Input: part model. Units: mm. Frame: model coordinates. Face numbers are marked on the shaded views. A direction names the side the tool comes from. Give positions to 0.01 mm unless a question says otherwise; leave off trailing zeros. Loops run counter-clockwise (first coordinate to the right, second up) from the corner with the lowest first, then second, coordinate; pieces in that order, holes last. Notation, with made-up numbers: (38.25, 3.25) - (43.25, 3.25) arc R16 ccw to (43.25, 14.25) - close; hole circle Ø5 at (39.25, 7). An arc over 180 degrees is marked (long way). One line per item, written item: value.
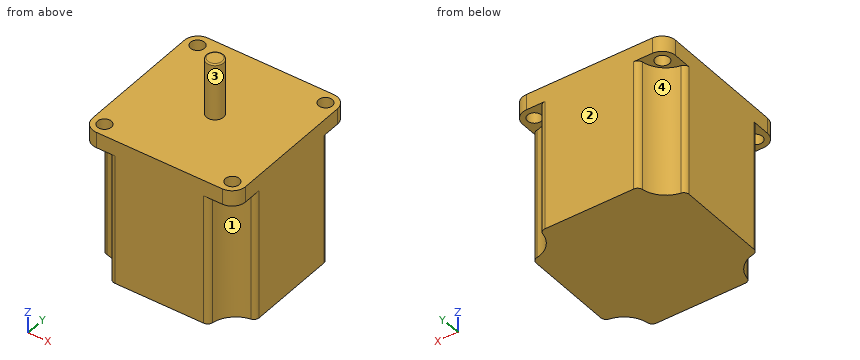
from build123d import *

# Parameters (mm, degrees)
ESQUISSE2_W             = 56.4
ESQUISSE2_H             = 56.4
BOSS_EXTRU_2_DEPTH      = 54
ESQUISSE3_R             = 2.55
ENL_V_MAT_EXTRU_1_DEPTH = 54
CONG_2_R                = 5
CONG_3_R                = 5
CONG_4_R                = 5
CONG_6_R                = 5
ESQUISSE4_R             = 2.55
ENL_V_MAT_EXTRU_2_DEPTH = 48.2
CONG_7_R                = 2
CONG_8_R                = 2
CONG_9_R                = 2
CONG_10_R               = 2
CONG_11_R               = 2
CONG_12_R               = 2
CONG_13_R               = 2
CONG_14_R               = 2
ESQUISSE5_R             = 3.175
BOSS_EXTRU_3_DEPTH      = 21
CONG_15_R               = 0.5


with BuildPart() as part:
    # Esquisse2 → Boss.-Extru.2 (new body)
    with BuildSketch(Plane.XY):
        Rectangle(ESQUISSE2_W, ESQUISSE2_H)
    extrude(amount=BOSS_EXTRU_2_DEPTH)

    # Esquisse3 → Enlèv. mat.-Extru.1 (cut)
    with BuildSketch(Plane.XY.offset(54)):
        with Locations((-23.57, 23.57)):
            Circle(ESQUISSE3_R)
        with Locations((23.57, 23.57)):
            Circle(ESQUISSE3_R)
        with Locations((23.57, -23.57)):
            Circle(ESQUISSE3_R)
        with Locations((-23.57, -23.57)):
            Circle(ESQUISSE3_R)
    extrude(amount=-ENL_V_MAT_EXTRU_1_DEPTH, mode=Mode.SUBTRACT)

    # Congé2
    cong_2_edges = [part.edges().sort_by_distance(p)[0] for p in [
        (28.2, 28.2, 27),
    ]]
    fillet(cong_2_edges, radius=CONG_2_R)

    # Congé3
    cong_3_edges = [part.edges().sort_by_distance(p)[0] for p in [
        (28.2, -28.2, 27),
    ]]
    fillet(cong_3_edges, radius=CONG_3_R)

    # Congé4
    cong_4_edges = [part.edges().sort_by_distance(p)[0] for p in [
        (-28.2, 28.2, 27),
    ]]
    fillet(cong_4_edges, radius=CONG_4_R)

    # Congé6
    cong_6_edges = [part.edges().sort_by_distance(p)[0] for p in [
        (-28.2, -28.2, 27),
    ]]
    fillet(cong_6_edges, radius=CONG_6_R)

    # Esquisse4 → Enlèv. mat.-Extru.2 (cut)
    with BuildSketch(Plane(origin=(0, 0, 0), x_dir=(-1, 0, 0), z_dir=(0, 0, -1))):
        with BuildLine():
            ThreePointArc((-18.2, -28.2), (-21.128932188, -21.128932188), (-28.2, -18.2))
            Line((-28.2, -18.2), (-28.2, -23.2))
            ThreePointArc((-28.2, -23.2), (-26.735533906, -26.735533906), (-23.2, -28.2))
            Line((-23.2, -28.2), (-18.2, -28.2))
        make_face()
        with Locations((-23.57, -23.57)):
            Circle(ESQUISSE4_R, mode=Mode.SUBTRACT)
        with BuildLine():
            Line((-28.2, 28.2), (-18.2, 28.2))
            ThreePointArc((-18.2, 28.2), (-21.128932188, 21.128932188), (-28.2, 18.2))
            Line((-28.2, 18.2), (-28.2, 28.2))
        make_face()
        with BuildLine():
            ThreePointArc((28.2, -18.2), (21.128932188, -21.128932188), (18.2, -28.2))
            Line((18.2, -28.2), (28.2, -28.2))
            Line((28.2, -28.2), (28.2, -18.2))
        make_face()
        with BuildLine():
            ThreePointArc((18.2, 28.2), (21.128932188, 21.128932188), (28.2, 18.2))
            Line((28.2, 18.2), (28.2, 28.2))
            Line((28.2, 28.2), (18.2, 28.2))
        make_face()
    extrude(amount=-ENL_V_MAT_EXTRU_2_DEPTH, mode=Mode.SUBTRACT)

    # Congé7
    cong_7_edges = [part.edges().sort_by_distance(p)[0] for p in [
        (18.2, 28.2, 24.1),
    ]]
    fillet(cong_7_edges, radius=CONG_7_R)

    # Congé8
    cong_8_edges = [part.edges().sort_by_distance(p)[0] for p in [
        (28.2, 18.2, 24.1),
    ]]
    fillet(cong_8_edges, radius=CONG_8_R)

    # Congé9
    cong_9_edges = [part.edges().sort_by_distance(p)[0] for p in [
        (-18.2, 28.2, 24.1),
    ]]
    fillet(cong_9_edges, radius=CONG_9_R)

    # Congé10
    cong_10_edges = [part.edges().sort_by_distance(p)[0] for p in [
        (-28.2, 18.2, 24.1),
    ]]
    fillet(cong_10_edges, radius=CONG_10_R)

    # Congé11
    cong_11_edges = [part.edges().sort_by_distance(p)[0] for p in [
        (-28.2, -18.2, 24.1),
    ]]
    fillet(cong_11_edges, radius=CONG_11_R)

    # Congé12
    cong_12_edges = [part.edges().sort_by_distance(p)[0] for p in [
        (-18.2, -28.2, 24.1),
    ]]
    fillet(cong_12_edges, radius=CONG_12_R)

    # Congé13
    cong_13_edges = [part.edges().sort_by_distance(p)[0] for p in [
        (18.2, -28.2, 24.1),
    ]]
    fillet(cong_13_edges, radius=CONG_13_R)

    # Congé14
    cong_14_edges = [part.edges().sort_by_distance(p)[0] for p in [
        (28.2, -18.2, 24.1),
    ]]
    fillet(cong_14_edges, radius=CONG_14_R)

    # Esquisse5 → Boss.-Extru.3 (add)
    with BuildSketch(Plane.XY.offset(54)):
        Circle(ESQUISSE5_R)
    extrude(amount=BOSS_EXTRU_3_DEPTH)

    # Congé15
    cong_15_edges = [part.edges().sort_by_distance(p)[0] for p in [
        (-3.175, 0, 75),
    ]]
    fillet(cong_15_edges, radius=CONG_15_R)


solid = part.part
Item 1: Access query for the marked faces 1, 2, 3 and 4. Directions: +Z, -Z, +X, -X, +Y, -Y. A direction counts if a zero-diameter tool reaches every point of the face in a straight line with its end or side. Return the directions, or none.
Verdict:
face 1: -Z, +X, -Y
face 2: +Z, -Z, +X, -X, +Y
face 3: +Z
face 4: -Z, -X, +Y
Item 2: Pin query (flat end, axial travel): P1, Ø3.5, axis at x = 23, y = 24.5, coming from the -Z side; P2, Ø5, axis at x = -17, y = -19, coming from the +Z side; P3, Ø3, axis at x = -23.57, y = 23.57, coming from the -Z side; P4, Ø5, axis at x = -4, z = 66, coming from the +Y side. Return the tip coordinate at first contact, or that it passes through.
Verdict:
P1: stops at z = 48.2
P2: stops at z = 54
P3: passes through
P4: stops at y = 2.8
Item 3: Section D-D, the plane x = 5.5. Output: boundary loops of the cut face in (y, z).
Verdict:
outline: (-28.2, 0) - (28.2, 0) - (28.2, 54) - (-28.2, 54) - close
Item 4: Section A-A, the plane z = 53. Output: boundary loops of the cut face in (x, y).
Verdict:
outline: (-28.2, -23.2) arc R5 ccw to (-23.2, -28.2) - (23.2, -28.2) arc R5 ccw to (28.2, -23.2) - (28.2, 23.2) arc R5 ccw to (23.2, 28.2) - (-23.2, 28.2) arc R5 ccw to (-28.2, 23.2) - close; hole circle Ø5.1 at (-23.57, -23.57); hole circle Ø5.1 at (-23.57, 23.57); hole circle Ø5.1 at (23.57, -23.57); hole circle Ø5.1 at (23.57, 23.57)
Item 5: Section B-B, the plane z = 7. Output: boundary loops of the cut face in (x, y), and give its area (3 significant figures).
Verdict:
outline: (-28.2, -16.37) arc R2 ccw to (-26.53, -18.34) arc R10 cw to (-18.34, -26.53) arc R2 ccw to (-16.37, -28.2) - (16.37, -28.2) arc R2 ccw to (18.34, -26.53) arc R10 cw to (26.53, -18.34) arc R2 ccw to (28.2, -16.37) - (28.2, 16.37) arc R2 ccw to (26.53, 18.34) arc R10 cw to (18.34, 26.53) arc R2 ccw to (16.37, 28.2) - (-16.37, 28.2) arc R2 ccw to (-18.34, 26.53) arc R10 cw to (-26.53, 18.34) arc R2 ccw to (-28.2, 16.37) - close
area: 2,860 mm^2
Item 6: Material intervals for L1, parallel to Y at x = 23.57, z = 49.5; L2, parallel to X at y = 23, z = 49; L3, parallel to Z at x = -24.5, y = -16.5, sorted ascending.
Verdict:
L1: y = -28.19 to -26.12, -21.02 to 21.02, 26.12 to 28.19
L2: x = -28.2 to -26.06, -21.08 to 21.08, 26.06 to 28.2
L3: z = 0 to 54
Item 7: Section C-C, the plane y = 0. Output: boundary loops of the cut face in (x, z) (3 decimals).
Verdict:
outline: (-28.2, 0) - (28.2, 0) - (28.2, 54) - (3.175, 54) - (3.175, 74.5) arc R0.5 ccw to (2.675, 75) - (-2.675, 75) arc R0.5 ccw to (-3.175, 74.5) - (-3.175, 54) - (-28.2, 54) - close
